Could you check a few things on this model? Use its own coordinates, in mm. Face numbers are marked on the shaded views. A direction names the side the tool comes from. Round coordinates to 2 decimals unless told otherwise and drop trailing zeros. Loops run counter-clockwise (first coordinate to the right, second up) from the corner with the lowest first, then second, coordinate; pieces in that order, holes last.
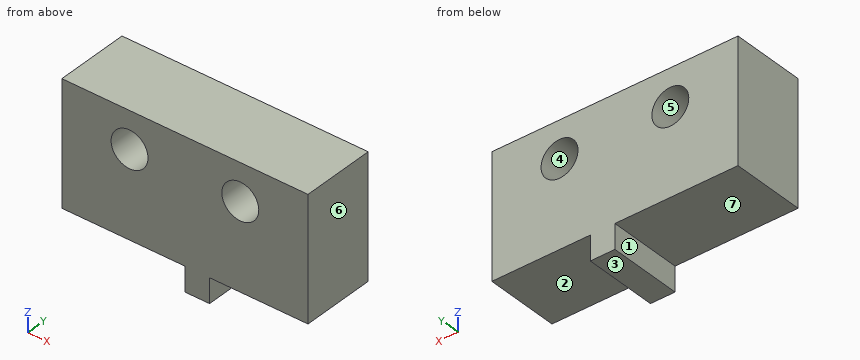
from build123d import *

# Parameters (mm, degrees)
CYLINDER033_R           = 1.5
CYLINDER033_DEPTH       = 10
ARRAY001016_Y_COUNT     = 2
ARRAY001016_Y_PITCH     = 9
BOX016_W                = 6
BOX016_H                = 20
BOX016_DEPTH            = 10
BOX017_W                = 6
BOX017_H                = 2
BOX017_DEPTH            = 2
BODY002_ROLL_ANGLE      = 180
BODY002_PLACEMENT_ANGLE = -90


with BuildPart() as end_stop_hole_array:
    # Cylinder033 → Cylinder033 (new body)
    with BuildSketch(Plane(origin=(-2, 5.5, 3), x_dir=(0, 0, -1), z_dir=(1, 0, 0))):
        Circle(CYLINDER033_R)
    extrude(amount=CYLINDER033_DEPTH)

    # Array001016 Y: end stop hole array ×2


with BuildPart() as end_stop_hole_array_1:
    add(end_stop_hole_array.part)
    with Locations(*[(0, i * ARRAY001016_Y_PITCH, 0) for i in range(1, ARRAY001016_Y_COUNT)]):
        add(end_stop_hole_array.part)


with BuildPart() as end_stop_body_cube:
    # Box016 → Box016 (new body)
    with BuildSketch(Plane.XY):
        with Locations((3, 10)):
            Rectangle(BOX016_W, BOX016_H)
    extrude(amount=BOX016_DEPTH)


with BuildPart() as end_stop_clone001:
    # Box017 → Box017 (new body)
    with BuildSketch(Plane(origin=(0, 8, 10), x_dir=(1, 0, 0), z_dir=(0, 0, 1))):
        with Locations((3, 1)):
            Rectangle(BOX017_W, BOX017_H)
    extrude(amount=BOX017_DEPTH)

    # Fusion013: union end stop body cube
    add(end_stop_body_cube.part)

    # Cut013: cut end stop hole array
    add(end_stop_hole_array_1.part, mode=Mode.SUBTRACT)


with BuildPart() as end_stop_clone001_1:
    # Body002 roll: moved
    add(end_stop_clone001.part.rotate(Axis((0, 0, 0), (1, 0, 0)), BODY002_ROLL_ANGLE))


with BuildPart() as end_stop_clone001_2:
    # Body002 placement: moved
    add(end_stop_clone001_1.part.moved(Location((111, 86.2588, 10.0341))).rotate(Axis((111, 86.2588, 10.0341), (0, 0, 1)), BODY002_PLACEMENT_ANGLE))


solid = end_stop_clone001_2.part
Item 1: We'd pull the mould along X, two halves only. Please class the marked faces 4, 5, 6 and 7: released by +X, released by -X, zero draft, split by the parting line, or undercut.
Results list:
face 4: undercut
face 5: undercut
face 6: released by +X
face 7: zero draft
Item 2: For the marked faces 1, 2 and 3, which set-ups out of +Z, -Z, +X, -X, +Y, -Y let a thin tool reach every point of the face, with its end or its side?
Results list:
face 1: -Z, -X, +Y, -Y
face 2: -Z, +X, +Y, -Y
face 3: -Z, +X, -X, +Y, -Y
Item 3: If I drill on line 1 along X through (y, z) = (82.9, 7); line 2 along X through (y, z) = (83.3, 8); line 3 along Z through (x, y) = (96.5, 81.5), over which ranges is the centre line in solid material (lowest first)?
Results list:
line 1: x = 91 to 95, 98 to 104, 107 to 111
line 2: x = 91 to 95.35, 97.65 to 104.35, 106.65 to 111
line 3: z = 0.03 to 5.53, 8.53 to 10.03
Item 4: If we section it at B-B, the plane y = 81.9: Please give me the cut outline in (x, z), then the cut area to 3 significant figures.
Results list:
outline: (91, 0.03) - (101, 0.03) - (101, -1.97) - (103, -1.97) - (103, 0.03) - (111, 0.03) - (111, 10.03) - (91, 10.03) - close; hole circle Ø3 at (96.5, 7.03); hole circle Ø3 at (105.5, 7.03)
area: 190 mm2
Item 5: If we section it at D-D, the plane z = -0.75: Please give me the cut outline in (x, y).
Results list:
outline: (101, 80.26) - (103, 80.26) - (103, 86.26) - (101, 86.26) - close
Item 6: If we section it at C-C, the plane z = 6: Please give me the cut outline in (x, y).
Results list:
outline: (91, 80.26) - (95.41, 80.26) - (95.41, 86.26) - (91, 86.26) - close; (97.59, 80.26) - (104.41, 80.26) - (104.41, 86.26) - (97.59, 86.26) - close; (106.59, 80.26) - (111, 80.26) - (111, 86.26) - (106.59, 86.26) - close
Item 7: Will these pins go through, and if not, where does the flat tip stop? pin 1 (5 mm diameter, centred on x = 96.5, z = 7.03, fed in from -Y); pin 2 (3 mm diameter, centred on x = 94, y = 83, fed in from -Z); pin 3 (0.6 mm diameter, centred on y = 83.5, z = -1, fed in from -X); pin 4 (1 mm diameter, centred on y = 82, z = -1, fed in from +X).
Results list:
pin 1: stops at y = 80.26
pin 2: stops at z = 0.03
pin 3: stops at x = 101
pin 4: stops at x = 103
Item 8: If we section it at A-A, the plane x = 105.5: Please give me the cut outline in (y, z), then the cut area to 3 significant figures.
Results list:
outline: (80.26, 0.03) - (86.26, 0.03) - (86.26, 5.53) - (80.26, 5.53) - close; (80.26, 8.53) - (86.26, 8.53) - (86.26, 10.03) - (80.26, 10.03) - close
area: 42.0 mm2
